The model under review builds one solid part; all positions refer to its coordinate system, in mm. A direction names the side the tool comes from. Coordinates: 2 decimals unless noted, no trailing zeros.
```python
from build123d import *

# Parameters (mm, degrees)
FORMED_WEB_DEPTH           = 10
EDGE_STIFFENING_LIPS_DEPTH = 214.533668262
WALL_MOUNT_HOLE_SKETCH_R   = 1.7
WALL_MOUNT_HOLES_DEPTH     = 2.4
COVER_MOUNT_HOLE_SKETCH_R  = 1.7
COVER_MOUNT_HOLE_DEPTH     = 2.4


with BuildPart() as part:
    # Formed Web Section Sketch → Formed Web (new body)
    with BuildSketch(Plane(origin=(185, 0, 0), x_dir=(0, 0, -1), z_dir=(1, 0, 0))):
        with BuildLine():
            Line((-22, 64), (-39.792590359, 64))
            ThreePointArc((-39.792590359, 64), (-42.163216653, 64.778178935), (-43.611457224, 66.809934512))
            Line((-43.611457224, 66.809934512), (-109.818866865, 279.266547538))
            ThreePointArc((-109.818866865, 279.266547538), (-109.954457451, 279.854727432), (-110, 280.456613027))
            Line((-110, 280.456613027), (-110, 290))
            Line((-110, 290), (-108, 290))
            Line((-108, 290), (-108, 280.456613027))
            ThreePointArc((-108, 280.456613027), (-107.977228725, 280.155670229), (-107.909433433, 279.861580283))
            Line((-107.909433433, 279.861580283), (-41.702023792, 67.404967256))
            ThreePointArc((-41.702023792, 67.404967256), (-40.977903506, 66.389089467), (-39.792590359, 66))
            Line((-39.792590359, 66), (-22, 66))
            Line((-22, 66), (-22, 64))
        make_face()
    extrude(amount=FORMED_WEB_DEPTH)

    # Edge Lip Sketch → Edge Stiffening Lips (add)
    with BuildSketch(Plane(origin=(0, 77.102620151, 24.02732814), x_dir=(-1, 0, 0), z_dir=(0, -0.9547167162884552, -0.297516372052681))):
        with BuildLine():
            Line((-181, -17.759537901), (-181, -11.759537901))
            Line((-181, -11.759537901), (-183, -11.759537901))
            Line((-183, -11.759537901), (-183, -17.759537901))
            ThreePointArc((-183, -17.759537901), (-183.585786438, -19.173751463), (-185, -19.759537901))
            Line((-185, -19.759537901), (-185.1, -19.759537901))
            Line((-185.1, -19.759537901), (-185.1, -21.759537901))
            Line((-185.1, -21.759537901), (-185, -21.759537901))
            ThreePointArc((-185, -21.759537901), (-182.171572875, -20.587965025), (-181, -17.759537901))
        make_face()
        with BuildLine():
            Line((-199, -17.759537901), (-199, -11.759537901))
            Line((-199, -11.759537901), (-197, -11.759537901))
            Line((-197, -11.759537901), (-197, -17.759537901))
            ThreePointArc((-197, -17.759537901), (-196.414213562, -19.173751463), (-195, -19.759537901))
            Line((-195, -19.759537901), (-194.9, -19.759537901))
            Line((-194.9, -19.759537901), (-194.9, -21.759537901))
            Line((-194.9, -21.759537901), (-195, -21.759537901))
            ThreePointArc((-195, -21.759537901), (-197.828427125, -20.587965025), (-199, -17.759537901))
        make_face()
    extrude(amount=-EDGE_STIFFENING_LIPS_DEPTH)

    # Wall Mount Hole Sketch → Wall Mount Holes (cut)
    with BuildSketch(Plane(origin=(0, 63.8, 0), x_dir=(-1, 0, 0), z_dir=(0, -1, 0))):
        with Locations(Location((-190, -29, 0), (0, 0, 90))):
            Circle(WALL_MOUNT_HOLE_SKETCH_R)
        with Locations(Location((-190, -36, 0), (0, 0, 90))):
            Circle(WALL_MOUNT_HOLE_SKETCH_R)
    extrude(amount=-WALL_MOUNT_HOLES_DEPTH, mode=Mode.SUBTRACT)

    # Cover Mount Hole Sketch → Cover Mount Hole (cut)
    with BuildSketch(Plane.XY.offset(107.8)):
        with Locations(Location((190, 285, 0), (0, 0, 180))):
            Circle(COVER_MOUNT_HOLE_SKETCH_R)
    extrude(amount=COVER_MOUNT_HOLE_DEPTH, mode=Mode.SUBTRACT)


solid = part.part
```
(1) Wall thickness on probe 1 along Z at (x, y) = (190, 64.55); probe 2 along Z at (x, y) = (190, 64.8); probe 3 along X at (y, z) = (285, 109.6): over which ranges is each line inside the solid? List them lowest first.
A:
probe 1: z = 22 to 27.3, 30.7 to 34.3, 37.7 to 41.82
probe 2: z = 22 to 27.3, 30.7 to 34.3, 37.7 to 42.19
probe 3: x = 185 to 188.3, 191.7 to 195
(2) Machinability: for faces 4 (the face through (196.43, 172.378, 73.785)), 5 (the face through (182.584, 72.137, 39.961)), 6 (the face through (190, 66, 31)), 7 (the face through (197.416, 72.137, 39.961)), which of the approach directions +Z, -Z, +X, -X, +Y, -Y give a long, thin tool a straight path to every point of the face, cutting with its end or side? Answer none if there is none.
A:
face 4: -Z, +Y
face 5: -Z, -X, -Y
face 6: -Z, +X, -X, +Y
face 7: -Z, +X, -Y
(3) For pin 1 Ø1.6 at (y, z) = (279.5, 108.5) entering from -X; pin 2 Ø5.5 at (x, y) = (190, 285) entering from -Z; pin 3 Ø1 at (x, z) = (193.5, 40.5) entering from -Y, all flat-tipped, find the tip position at first contact; note any pin that passes through.
A:
pin 1: stops at x = 185
pin 2: stops at z = 108
pin 3: stops at y = 64.01
(4) Draft analysis for pull direction X (two halves, no side actions). For faces 1 (the face through (185, 65.8, 34.2)), 2 (the face through (183, 174, 70)), 3 (the face through (182.584, 276.956, 103.788)), state which applies: released by +X, released by -X, zero draft, split by the parting line, or undercut.
A:
face 1: released by -X
face 2: undercut
face 3: zero draft
